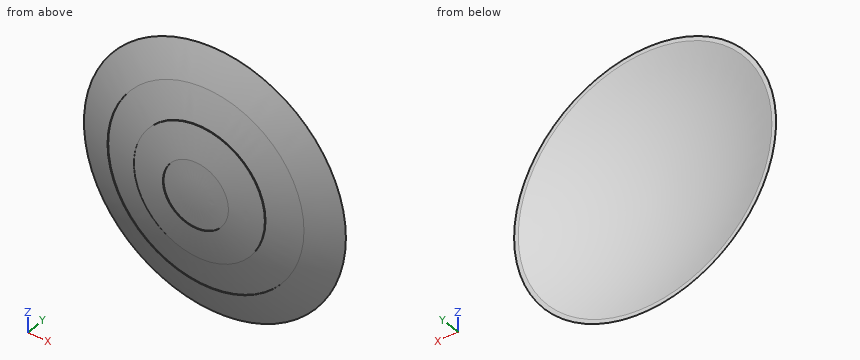
from build123d import *


with BuildPart() as f1:
    # F0 (on Top) → F1 (revolve)
    with BuildSketch(Plane.XY):
        with BuildLine():
            ThreePointArc((381, -1208.1740688431), (441.0588132701, -1187.5658734831), (500.0095805332, -1163.9742265188))
            Line((500.0095805332, -1163.9742265188), (491.9098723343, -1163.9742265188))
            ThreePointArc((491.9098723343, -1163.9742265188), (250.9534729382, -1238.4803902042), (0, -1263.65))
            Line((0, -1263.65), (0, -1266.825))
            ThreePointArc((0, -1266.825), (63.5801262199, -1265.2284964286), (127, -1260.4430096696))
            ThreePointArc((127, -1260.4430096696), (190.7453447969, -1252.3824472035), (254, -1241.1001493131))
            ThreePointArc((254, -1241.1001493131), (317.9265350577, -1226.2823080071), (381, -1208.1740688431))
        make_face()
        with BuildLine():
            Line((127, -1260.4430096696), (127, -1263.6340451254))
            ThreePointArc((127, -1263.6340451254), (190.7440888462, -1255.5941591813), (254, -1244.3407893339))
            Line((254, -1244.3407893339), (254, -1241.1001493131))
            ThreePointArc((254, -1241.1001493131), (190.7453447969, -1252.3824472035), (127, -1260.4430096696))
        make_face()
        with BuildLine():
            ThreePointArc((381, -1211.5027857995), (445.1348009163, -1189.4347434867), (508, -1163.9742265188))
            Line((508, -1163.9742265188), (500.0095805332, -1163.9742265188))
            ThreePointArc((500.0095805332, -1163.9742265188), (441.0588132701, -1187.5658734831), (381, -1208.1740688431))
            Line((381, -1208.1740688431), (381, -1211.5027857995))
        make_face()
    revolve(axis=Axis((0, -1266.825, 0), (0, -1, 0)))


solid = f1.part
Geometry check sheet. Reference: the model listing, model coordinates, mm. Coordinates: 2 decimals unless noted, no trailing zeros. Order: outer loops, then holes, each group sorted by start corner. A loop starts at its lowest first (then second) coordinate and runs counter-clockwise, first axis right, second up. Notation, with made-up numbers: M -25.75,-9.75 L -19.75,-9.75 A23 ccw -19.75,12.25 Z; hole C 60,18 d2. An arc over 180 degrees is marked long. Use CSV: the item, a comma, the result in double quotes.
Item 1: Cross-section at D-D on x = -180.5. Record the cut outline in (y, z).
Returned:
outline,"M -1244.34,-178.71 L -1241.1,-178.71 A1253.9 ccw -1208.17,-335.53 L -1211.5,-335.53 A1257.11 ccw -1163.97,-474.85 L -1163.97,-457.6 A1250.69 cw -1163.97,457.6 L -1163.97,474.85 A1257.11 ccw -1211.5,335.53 L -1208.17,335.53 A1253.9 ccw -1241.1,178.71 L -1244.34,178.71 A1257.11 ccw Z"
Item 2: Cross-section at B-B on z = 0. Record the cut outline in (x, y) (3 decimals), then the cut area to 3 significant figures.
Returned:
outline,"M -508,-1163.974 A1270 ccw -381,-1211.503 L -381,-1208.174 A1266.825 ccw -254,-1241.1 L -254,-1244.341 A1270 ccw -127,-1263.634 L -127,-1260.443 A1266.825 ccw 127,-1260.443 L 127,-1263.634 A1270 ccw 254,-1244.341 L 254,-1241.1 A1266.825 ccw 381,-1208.174 L 381,-1211.503 A1270 ccw 508,-1163.974 L 491.91,-1163.974 A1263.65 cw -491.91,-1163.974 Z"
area,"4,890 mm2"
Item 3: Cross-section at A-A on x = 0. Record the cut outline in (y, z) (3 decimals), then the cut area to 3 significant figures.
Returned:
outline,"M -1263.634,-127 A1270 ccw -1244.341,-254 L -1241.1,-254 A1266.825 ccw -1208.174,-381 L -1211.503,-381 A1270 ccw -1163.974,-508 L -1163.974,-491.91 A1263.65 cw -1163.974,491.91 L -1163.974,508 A1270 ccw -1211.503,381 L -1208.174,381 A1266.825 ccw -1241.1,254 L -1244.341,254 A1270 ccw -1263.634,127 L -1260.443,127 A1266.825 ccw -1260.443,-127 Z"
area,"4,890 mm2"
Item 4: Gauge pin test, flat ends, axial feed: pin 1 Ø2 at (x, z) = (-196.5, 242.5) entering from +Y; pin 2 Ø3 at (x, z) = (331, 57.5) entering from -Y. Record the tip position at first contact, or that the pin passes through.
Returned:
pin 1,"stops at y = -1224.24"
pin 2,"stops at y = -1221.88"
Item 5: Thickness scan on line 1 along Y through (x, z) = (190.5, -283.5); line 2 along Y through (x, z) = (210, 180). Record the ranges inside material, lowest first.
Returned:
line 1,"y = -1219.91 to -1216.61"
line 2,"y = -1236.26 to -1233.01"
Item 6: Cross-section at C-C on z = -273. Record the cut outline in (x, y).
Returned:
outline,"M -428.41,-1163.97 A1240.31 ccw -265.77,-1211.5 L -265.77,-1208.17 A1237.06 ccw 265.77,-1208.17 L 265.77,-1211.5 A1240.31 ccw 428.41,-1163.97 L 409.2,-1163.97 A1233.81 cw -409.2,-1163.97 Z"
